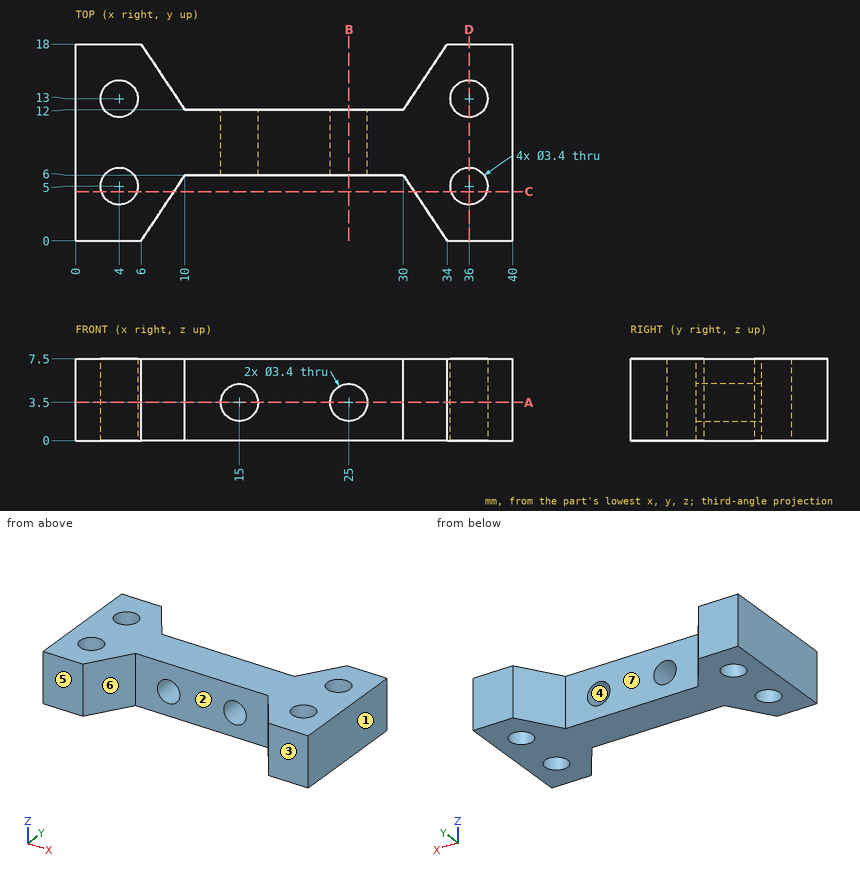
Geometry: see drawing. Coordinates: mm, zero at the bounding-box minimum. A direction names the side the tool comes from. Round coordinates to 2 decimals unless told otherwise and drop trailing zeros. Loops run counter-clockwise (first coordinate to the right, second up) from the corner with the lowest first, then second, coordinate; pieces in that order, holes last. Notation, with made-up numbers: M 42,61.5 L 81,61.5 A10 ccw 81,68.5 Z; hole C 16,-32.75 d7. An arc over 180 degrees is marked long. Use a Markdown table: item, result. Add a question column.
1. Cut plane B-B, the plane x = 25. Output: boundary loops of the cut face in (y, z).
2. Cut plane D-D, the plane x = 36. Output: boundary loops of the cut face in (y, z).
3. Contact query for flat-ended pins moving along their axis: pin 1 (4 mm diameter, centred on x = 28.5, z = 4.5, fed in from +Y); pin 2 (4.5 mm diameter, centred on x = 15, z = 3.5, fed in from +Y). Output: stop coordinate, or through.
4. Pull-direction query (X, two-part tool) for the marked faces 1, 2, 3 and 4; classes: +X half, -X half, draft (parallel to the pull), parting line (faces both ways), or undercut.
5. Cut plane A-A, the plane z = 3.5. Output: boundary loops of the cut face in (x, y), and give its area (3 significant figures).
6. Set-up query: the marked faces 5, 6 and 7. Return all of +Z, -Z, +X, -X, +Y, -Y with unobstructed straight access to the full face (end or side cutting, diameter ignored); none if empty.
7. Ray query, line 1 along Y through (x, z) = (4, 5); line 2 along X through (y, z) = (8.7, 3.5); line 3 along X through (y, z) = (14.5, 2.5). Return the intervals inside material, ascending. Write a range as [from, to].
8. Cut plane C-C, the plane y = 4.5. Output: boundary loops of the cut face in (x, z), and give its area (3 significant figures).
Solution:
| question | item | result |
|---|---|---|
| 1 | outline | M 6,0 L 12,0 L 12,1.8 L 6,1.8 Z; M 6,5.2 L 12,5.2 L 12,7.5 L 6,7.5 Z |
| 2 | outline | M 0,0 L 3.3,0 L 3.3,7.5 L 0,7.5 Z; M 6.7,0 L 11.3,0 L 11.3,7.5 L 6.7,7.5 Z; M 14.7,0 L 18,0 L 18,7.5 L 14.7,7.5 Z |
| 3 | pin 1 | stops at y = 12.75 |
| 3 | pin 2 | stops at y = 12 |
| 4 | face 1 | +X half |
| 4 | face 2 | undercut |
| 4 | face 3 | draft |
| 4 | face 4 | undercut |
| 5 | outline | M 0,0 L 6,0 L 10,6 L 13.3,6 L 13.3,12 L 10,12 L 6,18 L 0,18 Z; M 16.7,6 L 23.3,6 L 23.3,12 L 16.7,12 Z; M 26.7,6 L 30,6 L 34,0 L 40,0 L 40,18 L 34,18 L 30,12 L 26.7,12 Z; hole C 4,5 d3.4; hole C 4,13 d3.4; hole C 36,5 d3.4; hole C 36,13 d3.4 |
| 5 | area | 355 mm2 |
| 6 | face 5 | +Z, -Z, +X, -X, -Y |
| 6 | face 6 | +Z, -Z, -Y |
| 6 | face 7 | +Z, -Z, +Y |
| 7 | line 1 | y = [0, 3.3], [6.7, 11.3], [14.7, 18] |
| 7 | line 2 | x = [0, 13.3], [16.7, 23.3], [26.7, 40] |
| 7 | line 3 | x = [0, 3.2], [4.8, 8.33], [31.67, 35.2], [36.8, 40] |
| 8 | outline | M 0,0 L 2.38,0 L 2.38,7.5 L 0,7.5 Z; M 5.62,0 L 9,0 L 9,7.5 L 5.62,7.5 Z; M 31,0 L 34.38,0 L 34.38,7.5 L 31,7.5 Z; M 37.62,0 L 40,0 L 40,7.5 L 37.62,7.5 Z |
| 8 | area | 86.3 mm2 |
